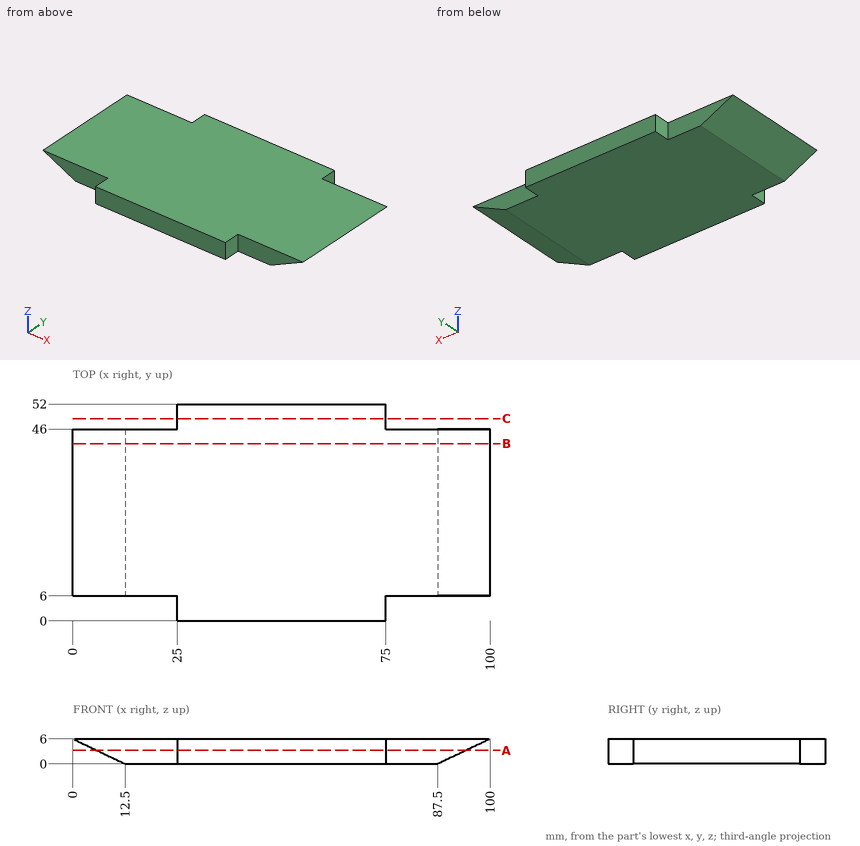
Check sheet for the drawn part. Datum: minimum x, y, z corner. Units: mm. Give positions to 0.01 mm unless a question says otherwise; leave off trailing zeros. Write each loop counter-clockwise with the first axis right and the second up, starting at its lowest first coordinate (ties: lowest second). Pieces come first, ordered by that corner, then holes.
(1) Cross-section at C-C (y = 48.5). Enter the section's corners in (x, z), plus the area to 3 significant figures.
(2) Cross-section at B-B (y = 42.5). Enter the section's corners in (x, z), plus the area to 3 significant figures.
(3) Gauge pin test, flat ends, axial feed: pin 1 (1.8 mm diameter, centred on y = 2, z = 4, fed in from +X); pin 2 (3 mm diameter, centred on x = 7.5, z = 4, fed in from +Y); pin 3 (3 mm diameter, centred on y = 3, z = 1.5, fed in from -X). Record the tip position at first contact, or that the pin passes through.
(4) Material ranges on line 1 (Y direction, x = 8, z = 4.5); line 2 (X direction, y = 25, z = 0.5); line 3 (X direction, y = 7, z = 2.5), recorded low to high.
(5) Cross-section at A-A (z = 3.25). Enter the section's corners in (x, y), plus the area to 3 significant figures.
Worked out:
1. outline: (25, 0) - (75, 0) - (75, 6) - (25, 6) - close
1. area: 300 mm2
2. outline: (0, 6) - (12.5, 0) - (87.5, 0) - (100, 6) - close
2. area: 525 mm2
3. pin 1: stops at x = 75
3. pin 2: stops at y = 46
3. pin 3: stops at x = 25
4. line 1: y = 6 to 46
4. line 2: x = 11.46 to 88.54
4. line 3: x = 7.29 to 92.71
5. outline: (5.73, 6) - (25, 6) - (25, 0) - (75, 0) - (75, 6) - (94.27, 6) - (94.27, 46) - (75, 46) - (75, 52) - (25, 52) - (25, 46) - (5.73, 46) - close
5. area: 4,140 mm2
